Work out the finished part from the listing and answer in its coordinate system (mm). Coordinates: 2 decimals unless noted, no trailing zeros. Order: outer loops, then holes, each group sorted by start corner. A loop starts at its lowest first (then second) coordinate and runs counter-clockwise, first axis right, second up.
1. The part is cut by section C-C, the plane y = -25. Give the vertices of the cut face in (x, z) (3 decimals).
2. The part is cut by section B-B, the plane z = 11. Give the vertices of the cut face in (x, y).
3. Find the intervals of material crossed by probe 1 along X at (y, z) = (-25, 2.85) (3 decimals); probe 2 along Y at (x, z) = (60, 2.05) (3 decimals); probe 3 along Z at (x, y) = (16.5, -35), in increasing order.
4. The part is cut by section D-D, the plane x = 8.5. Give the vertices of the cut face in (y, z), then the cut area to 3 significant figures.
5. The part is cut by section A-A, the plane x = 60. Give the vertices of the cut face in (y, z) (3 decimals), then the cut area to 3 significant figures.
6. Flat-ended cylindrical pins translate along their axes: pin 1 Ø12 at (x, y) = (29, -42) entering from +Z; pin 2 Ø2.5 at (y, z) = (-29, 10.5) entering from +X; pin 3 Ø3.5 at (x, z) = (6.5, 11) entering from -Y. Find the tip coordinate at first contact, or state that the pin passes through.
```python
from build123d import *

# Parameters (mm, degrees)
F0_W      = 120
F0_H      = 50
F1_DEPTH  = 8
F3_DEPTH  = 3
F5_DEPTH  = 25
F6_W      = 10
F6_H      = 3
F7_DEPTH  = 4.5
F8_SIZE   = 2
F9_W      = 0.5
F9_H      = 8.34277
F10_DEPTH = 1


with BuildPart() as f1:
    # F0 (on Top) → F1 (new body)
    with BuildSketch(Plane.XY):
        with Locations((60, -25)):
            Rectangle(F0_W, F0_H)
    extrude(amount=F1_DEPTH)

    # F2 (on face) → F3 (cut)
    with BuildSketch(Plane.XY.offset(8)):
        with BuildLine():
            Line((53.1, -14.45723), (53.1, -35.54277))
            ThreePointArc((53.1, -35.54277), (72.6, -25), (53.1, -14.45723))
        make_face()
    extrude(amount=-F3_DEPTH, mode=Mode.SUBTRACT)

    # F4 (on face) → F5 (cut)
    with BuildSketch(Plane.XY.offset(5)):
        with BuildLine():
            Line((55.1, -16.13966), (55.1, -33.86034))
            ThreePointArc((55.1, -33.86034), (70.125, -25), (55.1, -16.13966))
        make_face()
    extrude(amount=-F5_DEPTH, mode=Mode.SUBTRACT)

    # F6 (on face) → F7 (join)
    with BuildSketch(Plane.XY.offset(8)):
        with Locations((5, -21.3)):
            Rectangle(F6_W, F6_H)
        with Locations((5, -28.7)):
            Rectangle(F6_W, F6_H)
    extrude(amount=F7_DEPTH)

    # F8
    f8_edges = [f1.edges().sort_by_distance(p)[0] for p in [
        (120, -25, 8),
        (60, 0, 8),
        (60, -50, 8),
    ]]
    chamfer(f8_edges, length=F8_SIZE)

    # F9 (on face) → F10 (join)
    with BuildSketch(Plane.XY.offset(8)):
        with Locations((46.35, -18.628615)):
            Rectangle(F9_W, F9_H)
        with Locations((46.35, -31.371385)):
            Rectangle(F9_W, F9_H)
    extrude(amount=F10_DEPTH)


solid = f1.part
```
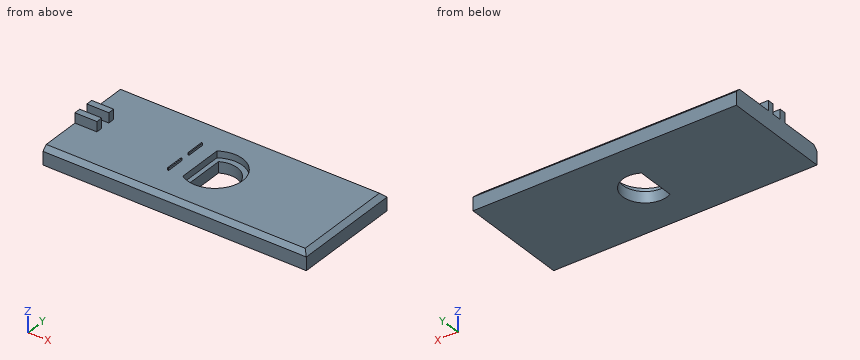
Geometry says:
1. outline: (0, 0) - (55.1, 0) - (55.1, 5) - (53.1, 5) - (53.1, 8) - (0, 8) - close; (70.125, 0) - (120, 0) - (120, 6) - (118, 8) - (72.6, 8) - (72.6, 5) - (70.125, 5) - close
2. outline: (0, -30.2) - (10, -30.2) - (10, -27.2) - (0, -27.2) - close; (0, -22.8) - (10, -22.8) - (10, -19.8) - (0, -19.8) - close
3. probe 1: x = 0 to 55.1, 70.125 to 120
3. probe 2: y = -50 to -35.125, -14.875 to 0
3. probe 3: z = 0 to 8
4. outline: (-50, 0) - (0, 0) - (0, 6) - (-2, 8) - (-19.8, 8) - (-19.8, 12.5) - (-22.8, 12.5) - (-22.8, 8) - (-27.2, 8) - (-27.2, 12.5) - (-30.2, 12.5) - (-30.2, 8) - (-48, 8) - (-50, 6) - close
4. area: 423 mm2
5. outline: (-50, 0) - (-35.125, 0) - (-35.125, 5) - (-37.6, 5) - (-37.6, 8) - (-48, 8) - (-50, 6) - close; (-14.875, 0) - (0, 0) - (0, 6) - (-2, 8) - (-12.4, 8) - (-12.4, 5) - (-14.875, 5) - close
5. area: 219 mm2
6. pin 1: stops at z = 8
6. pin 2: stops at x = 10
6. pin 3: stops at y = -30.2
